from build123d import *

# Parameters (mm, degrees)
SKETCH_1_R      = 3
EXTRUDE_1_DEPTH = 1.6
CHAMFER_1_SIZE  = 1.6
SKETCH_2_R      = 1.4
EXTRUDE_2_DEPTH = 26.6
CHAMFER_2_SIZE  = 0.2


with BuildPart() as part:
    # 草图1 → 凸台-拉伸1 (new body)
    with BuildSketch(Plane(origin=(0, 0, 0), x_dir=(1, 0, 0), z_dir=(0, 1, 0))):
        with Locations(Location((0, 0, 0), (0, 0, 270))):
            Circle(SKETCH_1_R)
        Polygon((0, -1.154700538), (1, -0.577350269), (1, 0.577350269), (0, 1.154700538), (-1, 0.577350269), (-1, -0.577350269), align=None, mode=Mode.SUBTRACT)
    extrude(amount=EXTRUDE_1_DEPTH)

    # 倒角1
    # the kernel refuses this chamfer: 1.6 mm, written as the material it takes off along each edge
    with BuildSketch(Plane(origin=(0, 1.6, 0), x_dir=(0, 0, 1), z_dir=(-1, 0, 0))) as chamfer_1_piece_1:
        Polygon((3, -CHAMFER_1_SIZE), (3 - CHAMFER_1_SIZE, 0), (3, 0), align=None)
    revolve(axis=Axis((0, 1.6, 0), (0, 1, 0)), mode=Mode.SUBTRACT)

    # 草图2 → 凸台-拉伸2 (add)
    with BuildSketch(Plane(origin=(0, 1.6, 0), x_dir=(1, 0, 0), z_dir=(0, 1, 0))):
        with Locations(Location((0, 0, 0), (0, 0, 270))):
            Circle(SKETCH_2_R)
    extrude(amount=EXTRUDE_2_DEPTH)

    # 倒角2
    chamfer_2_edges = [part.edges().sort_by_distance(p)[0] for p in [
        (0, 28.2, -1.4),
    ]]
    chamfer(chamfer_2_edges, length=CHAMFER_2_SIZE)


solid = part.part
For this review, take the finished solid that the model builds, in its own axes (mm). A direction names the side the tool comes from. Round coordinates to 2 decimals unless told otherwise and drop trailing zeros. Order: outer loops, then holes, each group sorted by start corner. A loop starts at its lowest first (then second) coordinate and runs counter-clockwise, first axis right, second up. Notation, with made-up numbers: M 36.25,-40 L 80.25,-40 A22 cw 80.25,-2 Z; hole C 21,-30 d8. An arc over 180 degrees is marked long. Use a Markdown table: item, result. Add a question column.
Item 1: Add section A-A, the plane z = 0. Give the boundary of the cut face in (x, y), then the cut area to 3 significant figures.
Item 2: Insertion check: pin 1 (2 mm diameter, centred on x = -2, y = 23.5, fed in from +Z); pin 2 (1 mm diameter, centred on x = 1, y = 11.5, fed in from +Z); pin 3 (3 mm diameter, centred on y = 19.5, z = 1, fed in from +X). Each pin has a flat end and moves straight along its axis. Give the tip position at first contact, or say it passes through.
Item 3: Add section B-B, the plane y = 6.5. Give the boundary of the cut face in (x, z).
Item 4: To check wall thickness, follow line 1 along X through (y, z) = (14, 0.05); line 2 along Y through (x, z) = (0.05, 0.75). State the ranges of each line that lie inside material, in increasing order.
Item 5: Mouldability with a two-part tool opening along Z and no side actions: class faces 3 (the cylindrical face through (0.06, 14.62, -1.4)), 4 (the flat face through (0.51, 0.79, -0.86)), 5 (the flat face through (-1.3, 0, 0)) as released by +Z, released by -Z, zero draft, split by the parting line, or undercut.
Item 6: Tool access review of faces 1 (the flat face through (-0.51, 0.79, 0.86)), 2 (the flat face through (0, 28.2, 0)): name each direction out of +Z, -Z, +X, -X, +Y, -Y from which nothing blocks a thin tool from reaching the whole face with its end or side.
Geometry results:
| question | item | result |
|---|---|---|
| 1 | outline | M -3,0 L -1,0 L -1,1.6 L 1,1.6 L 1,0 L 3,0 L 1.4,1.6 L 1.4,28 L 1.2,28.2 L -1.2,28.2 L -1.4,28 L -1.4,1.6 Z |
| 1 | area | 78.3 mm² |
| 2 | pin 1 | stops at z = 0.98 |
| 2 | pin 2 | stops at z = 1.31 |
| 2 | pin 3 | stops at x = 1.4 |
| 3 | outline | C 0,0 d2.8 |
| 4 | line 1 | x = -1.4 to 1.4 |
| 4 | line 2 | y = 1.6 to 28.2 |
| 5 | face 3 | split by the parting line |
| 5 | face 4 | undercut |
| 5 | face 5 | zero draft |
| 6 | face 1 | -Y |
| 6 | face 2 | +Z, -Z, +X, -X, +Y |
